```python
from build123d import *

# Parameters (mm, degrees)
SKETCH1_R           = 7.5
BOSS_EXTRUDE1_DEPTH = 30.15
SKETCH2_R           = 1.55
CUT_EXTRUDE1_DEPTH  = 30.15


with BuildPart() as part:
    # Sketch1 → Boss-Extrude1 (new body)
    with BuildSketch(Plane.XY):
        with BuildLine():
            Line((0, 0), (-34.1, 0))
            Line((-34.1, 0), (-34.1, 4))
            Line((-34.1, 4), (-27.05, 4))
            Line((-27.05, 4), (-27.05, 11))
            ThreePointArc((-27.05, 11), (-17.05, 21), (-7.05, 11))
            Line((-7.05, 11), (-7.05, 4))
            Line((-7.05, 4), (0, 4))
            Line((0, 4), (0, 0))
        make_face()
        with Locations((-17.05, 11)):
            Circle(SKETCH1_R, mode=Mode.SUBTRACT)
    extrude(amount=-BOSS_EXTRUDE1_DEPTH)

    # Sketch2 → Cut-Extrude1 (cut)
    with BuildSketch(Plane(origin=(0, 0, 0), x_dir=(-1, 0, 0), z_dir=(0, -1, 0))):
        with Locations(Location((29.05, 6, 0), (0, 0, 180))):
            Circle(SKETCH2_R)
        with Locations(Location((29.05, 24, 0), (0, 0, 180))):
            Circle(SKETCH2_R)
        with Locations(Location((5.05, 6, 0), (0, 0, 180))):
            Circle(SKETCH2_R)
        with Locations(Location((5.05, 24, 0), (0, 0, 180))):
            Circle(SKETCH2_R)
    extrude(amount=-CUT_EXTRUDE1_DEPTH, mode=Mode.SUBTRACT)


solid = part.part
```
Check sheet for the modelled part. Datum: model origin and axes. Units: mm. A direction names the side the tool comes from. Give positions to 0.01 mm unless a question says otherwise; leave off trailing zeros. Write each loop counter-clockwise with the first axis right and the second up, starting at its lowest first coordinate (ties: lowest second). Pieces come first, ordered by that corner, then holes.
Item 1: Access from +Z, -Z, +X, -X, +Y, -Y to the whole of each face (thin tool, end or side, straight path). Record for faces 1 (the face through (-17, 21, -15)), 2 (the face through (-31, 4, -15)), 3 (the face through (-4, 4, -15)).
Item 2: Draft check along Z on faces 4 (the face through (-6.6, 1.97, -5.93)), 5 (the face through (-21, 4, -30.15)), 6 (the face through (0, 2, -15)). Enter one of: released by +Z, released by -Z, zero draft, split by the parting line, or undercut.
Item 3: Cross-section at B-B (z = -6). Enter the section's corners in (x, y), and give its area (3 significant figures).
Item 4: Cross-section at D-D (x = -29.05). Enter the section's corners in (y, z), and give its area (3 significant figures).
Item 5: Cross-section at C-C (z = -12). Enter the section's corners in (x, y).
Item 6: Scan lines: L1, parallel to Z at x = -29.05, y = 1.3; L2, parallel to Y at x = -17.05, z = -11; L3, parallel to Y at x = -13, z = -4. Record each from-to range of solid material in increasing order.
Item 7: Gauge pin test, flat ends, axial feed: pin 1 (12 mm diameter, centred on x = -17.05, y = 11, fed in from -Z); pin 2 (2 mm diameter, centred on y = 14.5, z = -7.5, fed in from +X); pin 3 (4 mm diameter, centred on y = 11.5, z = -21.5, fed in from +X); pin 4 (3.5 mm diameter, centred on y = 7, z = -21.5, fed in from -X). Record the tip position at first contact, or that the pin passes through.
Item 8: Cross-section at A-A (x = -17.05). Enter the section's corners in (y, z), and give its area (3 significant figures).
Report:
1. face 1: +Z, -Z, +Y
1. face 2: +Z, -Z, -X, +Y
1. face 3: +Z, -Z, +X, +Y
2. face 4: undercut
2. face 5: released by -Z
2. face 6: zero draft
3. outline: (-34.1, 0) - (-30.6, 0) - (-30.6, 4) - (-34.1, 4) - close; (-27.5, 0) - (-6.6, 0) - (-6.6, 4) - (-7.05, 4) - (-7.05, 11) arc R10 ccw to (-27.05, 11) - (-27.05, 4) - (-27.5, 4) - close; (-3.5, 0) - (0, 0) - (0, 4) - (-3.5, 4) - close; hole circle Ø15 at (-17.05, 11)
3. area: 232 mm2
4. outline: (0, -30.15) - (4, -30.15) - (4, -25.55) - (0, -25.55) - close; (0, -22.45) - (4, -22.45) - (4, -7.55) - (0, -7.55) - close; (0, -4.45) - (4, -4.45) - (4, 0) - (0, 0) - close
4. area: 95.8 mm2
5. outline: (-34.1, 0) - (0, 0) - (0, 4) - (-7.05, 4) - (-7.05, 11) arc R10 ccw to (-27.05, 11) - (-27.05, 4) - (-34.1, 4) - close; hole circle Ø15 at (-17.05, 11)
6. L1: z = -30.15 to -25.55, -22.45 to -7.55, -4.45 to 0
6. L2: y = 0 to 3.5, 18.5 to 21
6. L3: y = 0 to 4.69, 17.31 to 20.14
7. pin 1: passes through
7. pin 2: stops at x = -7.37
7. pin 3: stops at x = -7.05
7. pin 4: stops at x = -27.05
8. outline: (0, -30.15) - (3.5, -30.15) - (3.5, 0) - (0, 0) - close; (18.5, -30.15) - (21, -30.15) - (21, 0) - (18.5, 0) - close
8. area: 181 mm2
